Geometry: final body of the model. Coordinates: model frame, mm. Coordinates: 2 decimals unless noted, no trailing zeros. Write each loop counter-clockwise with the first axis right and the second up, starting at its lowest first coordinate (ties: lowest second). Pieces come first, ordered by that corner, then holes. Notation, with made-up numbers: (27, -30) -> (83, -30) arc R26 cw to (83, -8) -> close; hole circle Ø7 at (31, -23.5). An arc over 180 degrees is marked (long way). One line per item, written item: value.
```python
from build123d import *

# Parameters (mm, degrees)
CROQUIS1_W                = 70
CROQUIS1_H                = 47.820638631
SALIENTE_EXTRUIR1_DEPTH   = 1
REDONDEO1_R               = 5
TALADRO_ROSCADO_M41_D     = 3.3
TALADRO_ROSCADO_M41_DEPTH = 11.5
TALADRO_ROSCADO_M41_TIP   = 0.991420021


with BuildPart() as part:
    # Croquis1 → Saliente-Extruir1 (new body)
    with BuildSketch(Plane(origin=(0, 0, 0), x_dir=(1, 0, 0), z_dir=(0, 1, 0))):
        with Locations((-28.897022241, -11.598967779)):
            Rectangle(CROQUIS1_W, CROQUIS1_H)
    extrude(amount=SALIENTE_EXTRUIR1_DEPTH)

    # Redondeo1
    redondeo1_edges = [part.edges().sort_by_distance(p)[0] for p in [
        (6.102977759, 0.5, 35.509287094),
        (-63.897022241, 0.5, 35.509287094),
        (-63.897022241, 0.5, -12.311351537),
        (6.102977759, 0.5, -12.311351537),
    ]]
    fillet(redondeo1_edges, radius=REDONDEO1_R)

    # Taladro roscado M41
    with Locations(Plane(origin=(0, 1, 0), x_dir=(1, 0, 0), z_dir=(0, 1, 0))):
        with Locations((-56.897022241, -11.598967779), (-0.897022241, -11.598967779)):
            Hole(TALADRO_ROSCADO_M41_D / 2, depth=TALADRO_ROSCADO_M41_DEPTH)
            with Locations((0, 0, -(TALADRO_ROSCADO_M41_DEPTH + TALADRO_ROSCADO_M41_TIP / 2))):  # 118° drill point
                Cone(0, TALADRO_ROSCADO_M41_D / 2, TALADRO_ROSCADO_M41_TIP, mode=Mode.SUBTRACT)


solid = part.part
```
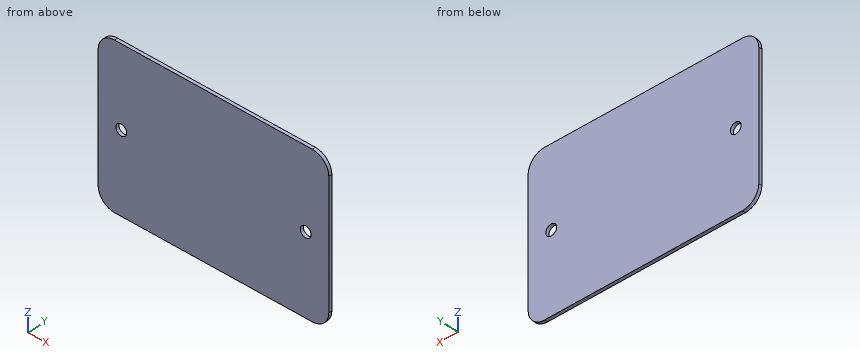
(1) Section B-B (x = -57.5). Return the cut outline in (y, z).
Responses:
outline: (0, -12.31) -> (1, -12.31) -> (1, 10.06) -> (0, 10.06) -> close; (0, 13.13) -> (1, 13.13) -> (1, 35.51) -> (0, 35.51) -> close
(2) Line query: line 1 (Z direction, x = -59, y = 0.95); line 2 (Z direction, x = -60, y = 0.1); line 3 (X direction, y = 0.3, z = 33). Output: solid intervals per line, ascending. Write a range as [from, to].
Responses:
line 1: z = [-12.31, 35.51]
line 2: z = [-12.19, 35.39]
line 3: x = [-63.23, 5.44]
(3) Section A-A (x = 0). Return the cut outline in (y, z).
Responses:
outline: (0, -12.31) -> (1, -12.31) -> (1, 10.21) -> (0, 10.21) -> close; (0, 12.98) -> (1, 12.98) -> (1, 35.51) -> (0, 35.51) -> close
(4) First-contact query: pin 1 (3 mm diameter, centred on x = -56.9, z = 11.6, fed in from -Y). Flat tip, straight axial feed; report the tip coordinate or a pass-through.
Responses:
pin 1: passes through
